The drawing under review shows one solid part. Ordinate dimensions are in mm from its lowest x, y, z. A direction names the side the tool comes from. Give positions to 0.01 mm unless a question says otherwise; leave off trailing zeros. Write each loop counter-clockwise with the first axis right and the second up, starting at its lowest first coordinate (ties: lowest second). Pieces come first, ordered by that corner, then holes. Notation, with made-up numbers: (26.5, 52) -> (75.5, 52) arc R13 ccw to (75.5, 69) -> close; hole circle Ø8 at (48, 60). An arc over 180 degrees is marked (long way). Answer as a JSON object with one key per item and string values.
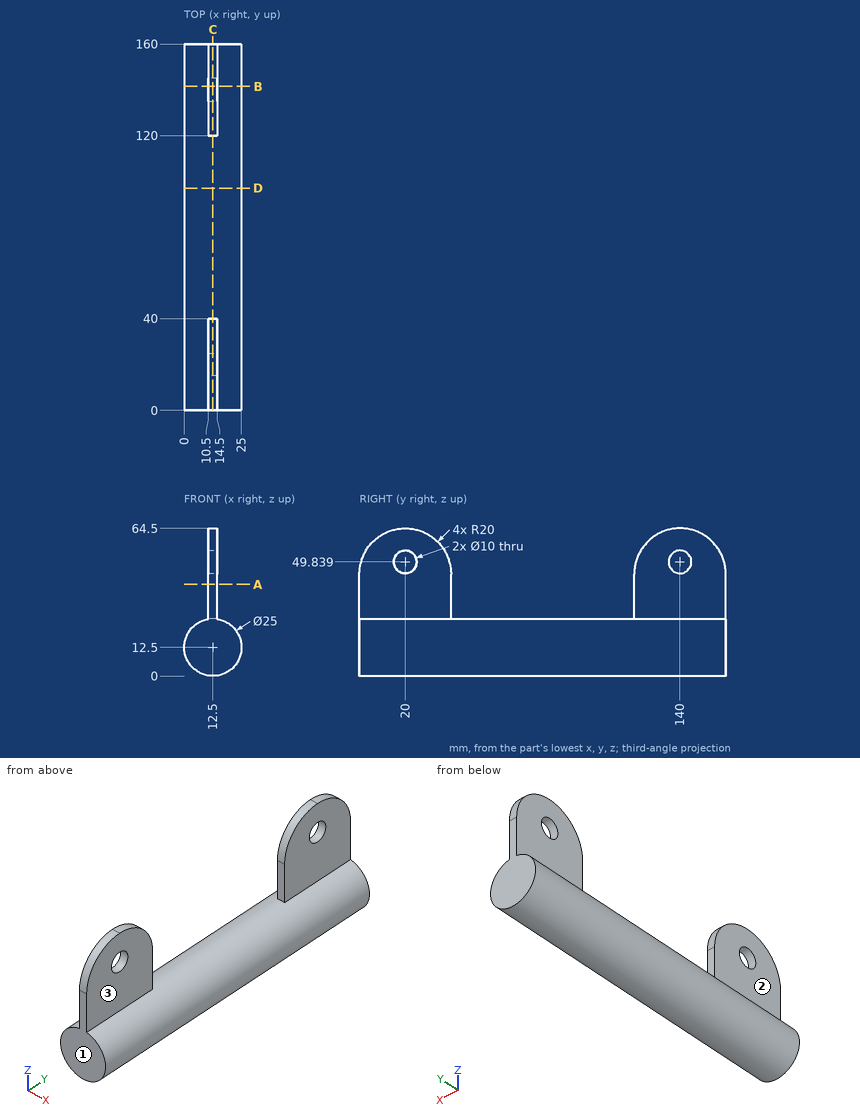
(1) Clearance check with flat-ended pins moving along their axes: pin 1 (1 mm diameter, centred on x = 11, z = 48.5, fed in from +Y); pin 2 (6 mm diameter, centred on x = 16, y = 58, fed in from -Z); pin 3 (1 mm diameter, centred on x = 3, y = 33.5, fed in from +Z) (1 decimal). State where each tip first meets the part, or that it passes through.
Here are the results:
{"pin 1": "stops at y = 159.69", "pin 2": "stops at z = 0.01", "pin 3": "stops at z = 21.2"}
(2) For line 1 along Z through (x, y) = (13.05, 20); line 2 along Y through (x, z) = (10.75, 33.5); line 3 along Z through (x, y) = (13.7, 140), list the stretches that pass through material, from the lowest coordinate up.
Here are the results:
{"line 1": "z = 0.01 to 44.84, 54.84 to 64.5", "line 2": "y = 0 to 40, 120 to 160", "line 3": "z = 0.06 to 44.84, 54.84 to 64.5"}
(3) We need section D-D, the plane y = 97. State the section outline as (x, z) points, then the cut area to 3 significant figures.
Here are the results:
{"outline": "circle Ø25 at (12.5, 12.5)", "area": "491 mm²"}
(4) We need section A-A, the plane z = 40. State the section outline as (x, y) points.
Here are the results:
{"outline": "(10.5, 0) -> (14.5, 0) -> (14.5, 40) -> (10.5, 40) -> close; (10.5, 120) -> (14.5, 120) -> (14.5, 160) -> (10.5, 160) -> close"}
(5) For the marked faces 1, 2 and 3, list the 3-axis set-ups (+Z, -Z, +X, -X, +Y, -Y) from which the entire face can be reached by the end or side of a thin tool; tool diameter is ignored.
Here are the results:
{"face 1": "+Z, -Z, +X, -X, -Y", "face 2": "+Z, -X, +Y, -Y", "face 3": "+Z, +X, +Y, -Y"}
(6) We need section B-B, the plane y = 141.5. State the section outline as (x, z) points.
Here are the results:
{"outline": "(10.5, 24.84) arc R12.5 ccw (long way) to (14.5, 24.84) -> (14.5, 45.07) -> (10.5, 45.07) -> close; (10.5, 54.61) -> (14.5, 54.61) -> (14.5, 64.44) -> (10.5, 64.44) -> close"}
(7) We need section C-C, the plane x = 12.5. Give the number of separate pieces and of enclosed holes in the cut face, then the cut area to 3 significant figures.
Here are the results:
{"separate pieces": "1", "enclosed holes": "2", "area": "6,660 mm²"}
